Source: CAD feature listing. Evaluate the final solid. Frame: model axes, mm. A direction names the side the tool comes from. Coordinates: 2 decimals unless noted, no trailing zeros. Loops run counter-clockwise (first coordinate to the right, second up) from the corner with the lowest first, then second, coordinate; pieces in that order, holes last.
```python
from build123d import *

# Parameters (mm, degrees)
BOSS_EXTRU_1_DEPTH = 7
D_GAGEMENT_M31_D   = 3.4
CONG_1_R           = 2


with BuildPart() as part:
    # Esquisse1 → Boss.-Extru.1 (new body)
    with BuildSketch(Plane(origin=(0, 0, 0), x_dir=(0, 0, -1), z_dir=(1, 0, 0))):
        Polygon((-37.5, 64.951905284), (-40.964101615, 62.951905284), (-24.964101615, 35.239092363), (-45.309401077, 0), (0, 0), (-2.309401077, 4), (-8.082903769, 4), (-23.232050808, 30.239092363), (-20.345299462, 35.239092363), align=None)
        Polygon((-38.381197846, 4), (-12.701705922, 4), (-25.541451884, 26.239092363), align=None, mode=Mode.SUBTRACT)
    extrude(amount=BOSS_EXTRU_1_DEPTH)

    # Dégagement M31 (through all)
    with Locations(Plane(origin=(0, 0, 0), x_dir=(-1, 0, 0), z_dir=(0, 0.5000000000000047, -0.866025403784436))):
        with Locations((-3.5, 71.2), (-3.5, 46)):
            Hole(D_GAGEMENT_M31_D / 2)

    # Congé1
    cong_1_edges = [part.edges().sort_by_distance(p)[0] for p in [
        (0, 63.951905284, 39.232050808),
        (3.5, 0, 0),
        (3.5, 0, 45.309401077),
        (3.5, 35.239092363, 24.964101615),
        (3.5, 35.239092363, 20.345299462),
        (3.5, 30.239092363, 23.232050808),
        (3.5, 4, 8.082903769),
        (3.5, 4, 2.309401077),
        (7, 63.951905284, 39.232050808),
        (3.5, 26.239092363, 25.541451884),
        (3.5, 4, 38.381197846),
        (3.5, 4, 12.701705922),
    ]]
    fillet(cong_1_edges, radius=CONG_1_R - 0.0001)  # a hair under: the kernel refuses the full size


solid = part.part
```
Q1. Section query C-C on y = 16. Return the cut outline in (x, z), then the cut area to 3 significant figures.
Q2. Section query B-B on z = 17.5. Return the cut outline in (x, y), then the cut area to 3 significant figures.
Q3. First-contact query: pin 1 Ø1 at (x, y) = (5.5, 46.5) entering from +Z; pin 2 Ø2 at (x, z) = (2, 25.5) entering from +Y; pin 3 Ø4 at (y, z) = (43, 22) entering from +X; pin 4 Ø4 at (x, y) = (1.5, 30) entering from +Z. Flat tips, straight axial feed; report the tip coordinate or a pass-through.
Q4. Material intervals for line 1 along Y through (x, z) = (6.75, 36); line 2 along Y through (x, z) = (2.5, 25); line 3 along Y through (x, z) = (6, 24.5), sorted ascending.
Q5. Reachability of faces 1 (the flat face through (3.45, 49.78, 33.36)), 2 (the flat face through (3.479, 63.966, 39.208)), 3 (the cylindrical face through (3.55, 4.97, 36.63)), 4 (the flat face through (3.45, 32.72, 21.8)), 5 (the cylindrical face through (3.549, 4.275, 7.941)) from +Z, -Z, +X, -X, +Y, -Y: full face, straight path, thin tool, end or side. Return the list, or none.
Q6. Section query A-A on x = 4. Count the separate pieces of the cut face and the enclosed holes in it, then the cut area to 3 significant figures.
Q7. Section query D-D on z = 30. Return the cut outline in (x, y).
Q8. Draft query along X for faces 6 (the flat face through (3, 0, 23)), 7 (the flat face through (7, 22.4, 22.8)), 8 (the cylindrical face through (3.13, 59.21, 36.53)). Return one class per face: released by +X, released by -X, zero draft, split by the parting line, or undercut.
Resolved:
1. outline: (0, 15.01) - (7, 15.01) - (7, 19.63) - (0, 19.63) - close; (0, 31.45) - (7, 31.45) - (7, 36.07) - (0, 36.07) - close
1. area: 64.7 mm2
2. outline: (0, 0) - (7, 0) - (7, 4) - (0, 4) - close; (0, 12.31) - (7, 12.31) - (7, 20.31) - (0, 20.31) - close
2. area: 84.0 mm2
3. pin 1: stops at z = 31.75
3. pin 2: stops at y = 45.9
3. pin 3: passes through
3. pin 4: stops at z = 29.14
4. line 1: y = 0 to 4.32, 8.12 to 16.12, 54.35 to 62.35
4. line 2: y = 0 to 4, 24.16 to 37.1, 40.27 to 43.3
4. line 3: y = 0 to 4, 23.95 to 42.44
5. face 1: +Z, +X, -X
5. face 2: +Z, +X, -X, +Y
5. face 3: +X, -X
5. face 4: -Z, +X, -X
5. face 5: -Z, +X, -X, +Y
6. separate pieces: 3
6. enclosed holes: 1
6. area: 538 mm2
7. outline: (0, 0) - (7, 0) - (7, 4) - (0, 4) - close; (0, 18.52) - (7, 18.52) - (7, 26.52) - (0, 26.52) - close; (0, 43.96) - (7, 43.96) - (7, 51.96) - (0, 51.96) - close
8. face 6: zero draft
8. face 7: released by +X
8. face 8: undercut
